from build123d import *

# Parameters (mm, degrees)
BOSS_EXTRUDE1_DEPTH = 75
SKETCH3_R           = 4
CUT_EXTRUDE1_DEPTH  = 65
BOSS_EXTRUDE2_DEPTH = 1
SKETCH5_R           = 12.5
CUT_EXTRUDE2_DEPTH  = 5
FILLET1_R           = 2


with BuildPart() as part:
    # Sketch1 → Boss-Extrude1 (new body)
    with BuildSketch(Plane.XY):
        with BuildLine():
            Line((-15, 10), (15, 10))
            Line((15, 10), (15, 5))
            ThreePointArc((15, 5), (9.643510109, 3.212979783), (5, 0))
            ThreePointArc((5, 0), (0, -5), (-5, 0))
            ThreePointArc((-5, 0), (-9.643510109, 3.212979783), (-15, 5))
            Line((-15, 5), (-15, 10))
        make_face()
    extrude(amount=-BOSS_EXTRUDE1_DEPTH)

    # Sketch3 → Cut-Extrude1 (cut)
    with BuildSketch(Plane(origin=(0, 0, -75), x_dir=(-1, 0, 0), z_dir=(0, 0, -1))):
        Circle(SKETCH3_R)
    extrude(amount=-CUT_EXTRUDE1_DEPTH, mode=Mode.SUBTRACT)

    # Sketch4 → Boss-Extrude2 (add)
    with BuildSketch(Plane(origin=(0, 10, 0), x_dir=(1, 0, 0), z_dir=(0, 1, 0))):
        with BuildLine():
            Line((-10, 63), (-10, 41))
            ThreePointArc((-10, 41), (0, 31), (10, 41))
            Line((10, 41), (10, 63))
            ThreePointArc((10, 63), (0, 73), (-10, 63))
        make_face()
    extrude(amount=BOSS_EXTRUDE2_DEPTH)

    # Sketch5 → Cut-Extrude2 (cut)
    with BuildSketch(Plane(origin=(0, 10, 0), x_dir=(1, 0, 0), z_dir=(0, 1, 0))):
        with Locations(Location((0, 15, 0), (0, 0, 180))):
            Circle(SKETCH5_R)
    extrude(amount=-CUT_EXTRUDE2_DEPTH, mode=Mode.SUBTRACT)

    # Fillet1
    fillet1_edges = [part.edges().sort_by_distance(p)[0] for p in [
        (-15, 10, -37.5),
        (15, 10, -37.5),
        (0, 10, -75),
        (0, 10, 0),
    ]]
    fillet(fillet1_edges, radius=FILLET1_R - 0.0001)  # a hair under: the kernel refuses the full size


solid = part.part
Geometry check sheet. Reference: the model listing, model coordinates, mm. A direction names the side the tool comes from. Coordinates: 2 decimals unless noted, no trailing zeros. Write each loop counter-clockwise with the first axis right and the second up, starting at its lowest first coordinate (ties: lowest second). Pieces come first, ordered by that corner, then holes. Notation, with made-up numbers: (65, 47) -> (95, 47) arc R16 ccw to (95, 52) -> close; hole circle Ø1 at (83.25, 2.5). An arc over 180 degrees is marked (long way). One line per question, with ' | ' between items.
1. Cross-section at D-D on y = 8.75. Record the cut outline in (x, z).
Answers:
outline: (-14.85, -74.85) -> (14.85, -74.85) -> (14.85, -0.15) -> (-14.85, -0.15) -> close; hole circle Ø25 at (0, -15)
2. Cross-section at C-C on x = 11.5. Record the cut outline in (y, z).
Answers:
outline: (4.03, -75) -> (8, -75) arc R2 ccw to (10, -73) -> (10, -19.9) -> (5, -19.9) -> (5, -10.1) -> (10, -10.1) -> (10, -2) arc R2 ccw to (8, 0) -> (4.03, 0) -> close
3. Set-up check for faces 5 (the flat face through (0, 5, -15)), 6 (the flat face through (0, 0, -10)), 7 (the cylindrical face through (-0.2, 10.5, -31)): record each of +Z, -Z, +X, -X, +Y, -Y from which the full face is reachable in a straight line by a thin tool's end or side.
Answers:
face 5: +Y | face 6: -Z | face 7: +Z, +Y
4. Draft check along X on faces 1 (the cylindrical face through (0.2, 10.5, -73)), 2 (the flat face through (-15, 6, -37)), 3 (the cylindrical face through (2.71, 7.535, -27.203)), 4 (the cylindrical face through (0.21, 9.43, -0.6)). Enter one of: +X half, -X half, draft (parallel to the pull), parting line (faces both ways), or undercut.
Answers:
face 1: parting line | face 2: -X half | face 3: undercut | face 4: draft
5. Cross-section at A-A on z = -61. Record the cut outline in (x, y).
Answers:
outline: (-15, 5) arc R20 cw to (-5, 0) arc R5 ccw to (5, 0) arc R20 cw to (15, 5) -> (15, 8) arc R2 ccw to (13, 10) -> (10, 10) -> (10, 11) -> (-10, 11) -> (-10, 10) -> (-13, 10) arc R2 ccw to (-15, 8) -> close; hole circle Ø8 at (0, 0)
6. Thickness scan on probe 1 along Y at (x, z) = (0, -36.5); probe 2 along Y at (x, z) = (0, -23.5); probe 3 along Z at (x, y) = (1.25, 3.5). Record the ranges inside material, lowest first. Write a range as from..to.
Answers:
probe 1: y = -5..-4, 4..11 | probe 2: y = -5..-4, 4..5 | probe 3: z = -10..0
7. Cross-section at B-B on y = 2.75. Record the cut outline in (x, z), and give its area (3 significant figures).
Answers:
outline: (-8.77, -75) -> (-2.9, -75) -> (-2.9, -10) -> (2.9, -10) -> (2.9, -75) -> (8.77, -75) -> (8.77, 0) -> (-8.77, 0) -> close | area: 938 mm²
8. Depth check by flat-ended pin: pin 1 Ø2 at (x, y) = (7.5, 3) entering from +Z; pin 2 Ø3 at (x, z) = (-8, -20) entering from +Y; pin 3 Ø1.5 at (y, z) = (1, -20.5) entering from +X; pin 4 Ø1 at (x, z) = (3, -21.5) entering from -Y. Enter the tip coordinate at first touch or a pass-through.
Answers:
pin 1: stops at z = 0 | pin 2: stops at y = 5 | pin 3: stops at x = 7.18 | pin 4: stops at y = -4.33
